The listing builds one solid part. Answer for the finished solid, in the listing's coordinates (mm). A direction names the side the tool comes from. Coordinates: 2 decimals unless noted, no trailing zeros. Loops run counter-clockwise (first coordinate to the right, second up) from the corner with the lowest first, then second, coordinate; pieces in that order, holes last. Notation, with made-up numbers: (0, 23) - (56, 23) arc R23 cw to (56, 45) - close; hole circle Ø9 at (-14, 11). An arc over 180 degrees is marked (long way). Return JSON: item names as keys, results as strings. Group by question number.
1. Find the intervals of material crossed by line 1 along Z through (x, y) = (54, 3.75); line 2 along Y through (x, z) = (57.25, 3); line 3 along X through (y, z) = (1, 3.25), in increasing order.
2. Section B-B (y = 8.75) is taken. Write down the section's boundary in (x, z).
3. This flat-tipped pin is pushed along its axis until it touches: P1, Ø1.1, axis at x = 53.5, z = 5, coming from the -Y side. Where does it stop, or does it pass through?
4. The mould has two halves that part along X. Classify faces 5 (the face through (54, 6, 1.5)), 6 (the face through (54.831, 3.584, 2.903)), 7 (the face through (50.5, 6, 4)): pulls with the +X half, pulls with the -X half, needs draft (parallel to the pull), parting line crosses it, or undercut.
5. Which of the six approach directions +Z, -Z, +X, -X, +Y, -Y give full straight-line access (tool end or side, diameter ignored) to faces 1 (the face through (54, 9.5, 5)), 2 (the face through (50.8, 0, 4)), 3 (the face through (57.2, 0, 4.3)), 4 (the face through (56, -2.5, 4))?
6. Section A-A (z = 4.5) is taken. Write down the section's boundary in (x, y).
```python
from build123d import *

# Parameters (mm, degrees)
CYLINDER002_R     = 1.8
CYLINDER002_DEPTH = 12
CYLINDER001_R     = 3
CYLINDER001_DEPTH = 2.5
BOX054_W          = 7
BOX054_H          = 12.5
BOX054_DEPTH      = 6
FILLET010_R       = 0.3


with BuildPart() as cylinder:
    # Cylinder002 → Cylinder002 (new body)
    with BuildSketch(Plane(origin=(0, 9.5, 3), x_dir=(1, 0, 0), z_dir=(0, -1, 0))):
        Circle(CYLINDER002_R)
    extrude(amount=CYLINDER002_DEPTH)


with BuildPart() as cylinder001:
    # Cylinder001 → Cylinder001 (new body)
    with BuildSketch(Plane(origin=(0, 0, 3), x_dir=(1, 0, 0), z_dir=(0, -1, 0))):
        Circle(CYLINDER001_R)
    extrude(amount=CYLINDER001_DEPTH)


with BuildPart() as phone_socket_audio_video:
    # Box054 → Box054 (new body)
    with BuildSketch(Plane(origin=(-3.5, 0, 0), x_dir=(1, 0, 0), z_dir=(0, 0, 1))):
        with Locations((3.5, 6.25)):
            Rectangle(BOX054_W, BOX054_H)
    extrude(amount=BOX054_DEPTH)

    # Fusion043: union Cylinder001
    add(cylinder001.part)

    # Cut010: cut Cylinder
    add(cylinder.part, mode=Mode.SUBTRACT)

    # Fillet010
    fillet010_edges = [phone_socket_audio_video.edges().sort_by_distance(p)[0] for p in [
        (-3, -2.5, 3),
    ]]
    fillet(fillet010_edges, radius=FILLET010_R)


with BuildPart() as phone_socket_audio_video_1:
    # Fillet010 placement: moved
    add(phone_socket_audio_video.part.moved(Location((54, 0, 1.5))))


solid = phone_socket_audio_video_1.part
```
The answers:
{
 "1": {"line 1": "z = 1.5 to 2.7, 6.3 to 7.5", "line 2": "y = 0 to 12.5", "line 3": "x = 50.5 to 52.7, 55.3 to 57.5"},
 "2": {"outline": "(50.5, 1.5) - (57.5, 1.5) - (57.5, 7.5) - (50.5, 7.5) - close; hole circle Ø3.6 at (54, 4.5)"},
 "3": {"P1": "stops at y = 9.5"},
 "4": {"face 5": "needs draft", "face 6": "undercut", "face 7": "pulls with the -X half"},
 "5": {"face 1": "-Y", "face 2": "-X, -Y", "face 3": "+X, -Y", "face 4": "+Z, -Z, +X, -X, -Y"},
 "6": {"outline": "(50.5, 0) - (51, 0) - (51, -2.2) arc R0.3 ccw to (51.3, -2.5) - (52.2, -2.5) - (52.2, 9.5) - (55.8, 9.5) - (55.8, -2.5) - (56.7, -2.5) arc R0.3 ccw to (57, -2.2) - (57, 0) - (57.5, 0) - (57.5, 12.5) - (50.5, 12.5) - close"}
}
